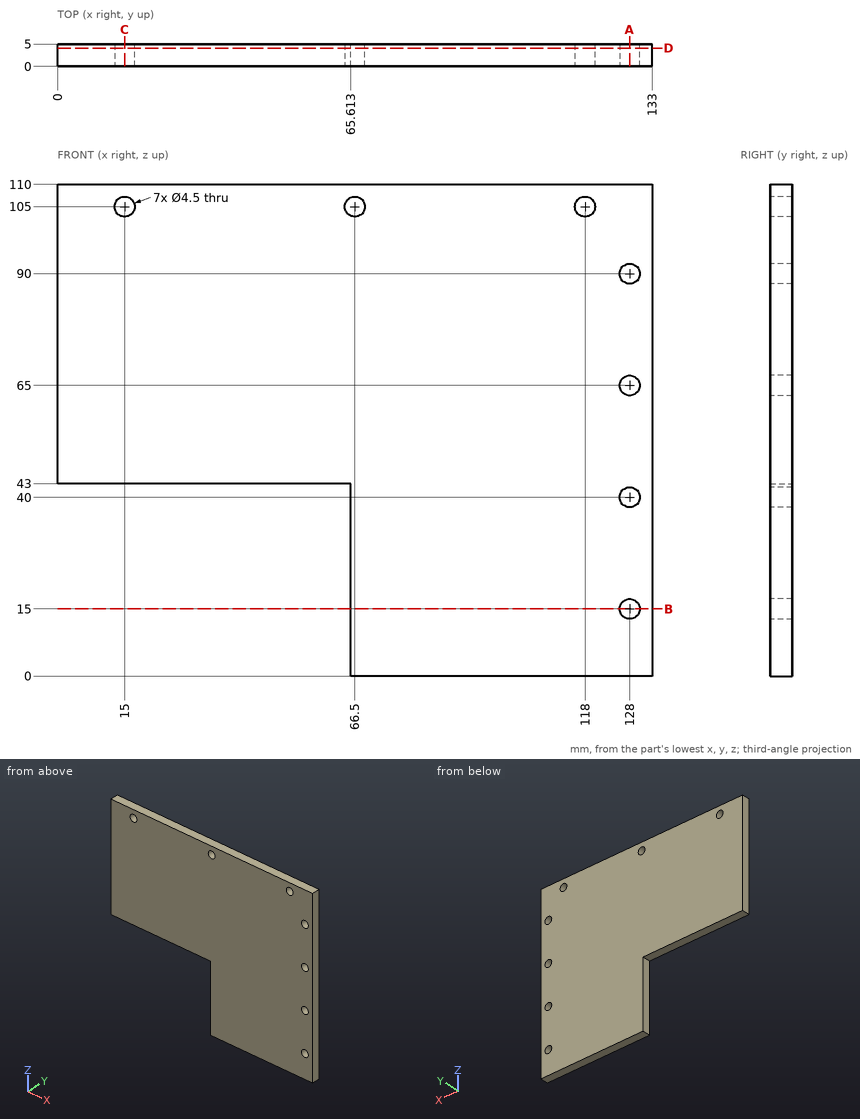
Design review of the part shown in the three views and the two pictorial views. Dimensions are in mm from the part's minimum x, y and z. Round coordinates to 2 decimals unless told otherwise and drop trailing zeros. Write each loop counter-clockwise with the first axis right and the second up, starting at its lowest first coordinate (ties: lowest second). Pieces come first, ordered by that corner, then holes. Notation, with made-up numbers: (7, 5.5) - (60, 5.5) arc R20 cw to (60, 25.5) - close; hole circle Ø9 at (2.25, -8.5). An arc over 180 degrees is marked (long way). Write item = value, one per line. Start each with the question number.
1. Consider section D-D on y = 4.1. State the section outline as (x, z) points.
2. Wall thickness on L1, parallel to Z at x = 128, y = 3.9; L2, parallel to X at y = 3.2, z = 105; L3, parallel to X at y = 1.3, z = 15: over which ranges is each line inside the solid? List them lowest first.
3. Consider section A-A on x = 128. State the section outline as (y, z) points, plus the area to 3 significant figures.
4. Consider section B-B on z = 15. State the section outline as (x, y) points.
5. Consider section C-C on x = 15. State the section outline as (y, z) points.
6. For pin 1 Ø4 at (x, z) = (118, 105) entering from +Y; pin 2 Ø1.5 at (y, z) = (1.5, 19.5) entering from -X, all flat-tipped, find the tip position at first contact; note any pin that passes through.
Evaluation:
q1.outline = (0, 43) - (65.61, 43) - (65.61, 0) - (133, 0) - (133, 110) - (0, 110) - close; hole circle Ø4.5 at (15, 105); hole circle Ø4.5 at (66.5, 105); hole circle Ø4.5 at (118, 105); hole circle Ø4.5 at (128, 15); hole circle Ø4.5 at (128, 40); hole circle Ø4.5 at (128, 65); hole circle Ø4.5 at (128, 90)
q2.L1 = 0 to 12.75, 17.25 to 37.75, 42.25 to 62.75, 67.25 to 87.75, 92.25 to 110
q2.L2 = 0 to 12.75, 17.25 to 64.25, 68.75 to 115.75, 120.25 to 133
q2.L3 = 65.61 to 125.75, 130.25 to 133
q3.outline = (0, 0) - (5, 0) - (5, 12.75) - (0, 12.75) - close; (0, 17.25) - (5, 17.25) - (5, 37.75) - (0, 37.75) - close; (0, 42.25) - (5, 42.25) - (5, 62.75) - (0, 62.75) - close; (0, 67.25) - (5, 67.25) - (5, 87.75) - (0, 87.75) - close; (0, 92.25) - (5, 92.25) - (5, 110) - (0, 110) - close
q3.area = 460 mm2
q4.outline = (65.61, 0) - (125.75, 0) - (125.75, 5) - (65.61, 5) - close; (130.25, 0) - (133, 0) - (133, 5) - (130.25, 5) - close
q5.outline = (0, 43) - (5, 43) - (5, 102.75) - (0, 102.75) - close; (0, 107.25) - (5, 107.25) - (5, 110) - (0, 110) - close
q6.pin_1 = through
q6.pin_2 = 65.61
